Can you work these out from the model? Positions are in its coordinate system, mm. A direction names the side the tool comes from. Round coordinates to 2 decimals unless told otherwise and drop trailing zeros. Order: outer loops, then holes, each group sorted by start corner. A loop starts at its lowest first (then second) coordinate and runs counter-clockwise, first axis right, second up. Notation, with made-up numbers: (14, 23) -> (22, 23) arc R22 cw to (22, 58) -> close; hole circle Ø5 at (67, -35). An arc over 180 degrees is marked (long way). One line per item, written item: value.
```python
from build123d import *

# Parameters (mm, degrees)
BOSS_EXTRUDE1_DEPTH = 27
SKETCH3_R           = 1.7
CUT_EXTRUDE2_DEPTH  = 35.322004603
SKETCH4_W           = 10
SKETCH4_H           = 20
CUT_EXTRUDE3_DEPTH  = 1
SKETCH5_R           = 2.25
CUT_EXTRUDE4_DEPTH  = 36.057096286
BOSS_EXTRUDE2_DEPTH = 3
SKETCH7_W           = 7
SKETCH7_H           = 3
BOSS_EXTRUDE3_DEPTH = 27
SKETCH8_R           = 2.25
CUT_EXTRUDE5_DEPTH  = 59.446556785
SKETCH9_R           = 4.25
CUT_EXTRUDE6_DEPTH  = 59.446556785
SKETCH11_W          = 16
SKETCH11_H          = 9
CUT_EXTRUDE7_DEPTH  = 59.446556785


with BuildPart() as part:
    # Sketch1 → Boss-Extrude1 (new body)
    with BuildSketch(Plane.XY):
        Polygon((0, 0), (0, 20), (3, 20), (3, 0), (10, 0), (10, -3), (0, -3), align=None)
    extrude(amount=BOSS_EXTRUDE1_DEPTH)

    # Sketch3 → Cut-Extrude2 (cut, through all)
    with BuildSketch(Plane(origin=(3, 0, 0), x_dir=(0, 0, -1), z_dir=(1, 0, 0))):
        with Locations(Location((-22, 14.85, 0), (0, 0, 90))):
            Circle(SKETCH3_R)
        with Locations(Location((-3, 14.85, 0), (0, 0, 90))):
            Circle(SKETCH3_R)
    extrude(amount=-CUT_EXTRUDE2_DEPTH, mode=Mode.SUBTRACT)

    # Sketch4 → Cut-Extrude3 (cut)
    with BuildSketch(Plane(origin=(3, 0, 0), x_dir=(0, 0, -1), z_dir=(1, 0, 0))):
        with Locations((-12.5, 10)):
            Rectangle(SKETCH4_W, SKETCH4_H)
    extrude(amount=-CUT_EXTRUDE3_DEPTH, mode=Mode.SUBTRACT)

    # Sketch5 → Cut-Extrude4 (cut, through all)
    with BuildSketch(Plane(origin=(0, 0, 0), x_dir=(1, 0, 0), z_dir=(0, 1, 0))):
        with Locations(Location((6.5, -9, 0), (0, 0, 270))):
            Circle(SKETCH5_R)
    extrude(amount=-CUT_EXTRUDE4_DEPTH, mode=Mode.SUBTRACT)

    # Sketch6 → Boss-Extrude2 (add)
    with BuildSketch(Plane.ZY):
        Polygon((27, 9), (54, 0), (54, -3), (27, -3), align=None)
    extrude(amount=-BOSS_EXTRUDE2_DEPTH)

    # Sketch7 → Boss-Extrude3 (add)
    with BuildSketch(Plane.XY.offset(27)):
        with Locations((6.5, -1.5)):
            Rectangle(SKETCH7_W, SKETCH7_H)
    extrude(amount=BOSS_EXTRUDE3_DEPTH)

    # Sketch8 → Cut-Extrude5 (cut, through all)
    with BuildSketch(Plane(origin=(0, 0, 0), x_dir=(1, 0, 0), z_dir=(0, 1, 0))):
        with Locations(Location((6.5, -39, 0), (0, 0, 270))):
            Circle(SKETCH8_R)
    extrude(amount=-CUT_EXTRUDE5_DEPTH, mode=Mode.SUBTRACT)

    # Sketch9 → Cut-Extrude6 (cut, through all)
    with BuildSketch(Plane(origin=(0, 0, 0), x_dir=(1, 0, 0), z_dir=(0, 1, 0))):
        with Locations((6.5, -39)):
            Circle(SKETCH9_R)
    extrude(amount=CUT_EXTRUDE6_DEPTH, mode=Mode.SUBTRACT)

    # Sketch11 → Cut-Extrude7 (cut, through all)
    with BuildSketch(Plane(origin=(10, 0, 0), x_dir=(0, 0, -1), z_dir=(1, 0, 0))):
        with Locations((-8, 1.5)):
            Rectangle(SKETCH11_W, SKETCH11_H)
    extrude(amount=-CUT_EXTRUDE7_DEPTH, mode=Mode.SUBTRACT)


solid = part.part
```
Q1. I want a section at B-B on z = 3. List the corners of the cut face in (x, y) for me.
Answers below:
outline: (0, 6) -> (3, 6) -> (3, 13.15) -> (0, 13.15) -> close; (0, 16.55) -> (3, 16.55) -> (3, 20) -> (0, 20) -> close
Q2. I want a section at C-C on x = 6.5. List the corners of the cut face in (y, z) for me, plus the area to 4 significant figures.
Answers below:
outline: (-3, 16) -> (0, 16) -> (0, 36.75) -> (-3, 36.75) -> close; (-3, 41.25) -> (0, 41.25) -> (0, 54) -> (-3, 54) -> close
area: 100.5 mm^2
Q3. Please list where these lines run through material, in increasing order: line 1 along Z through (x, y) = (1.9, 14.85); line 2 along X through (y, z) = (-1.75, 39); line 3 along Z through (x, y) = (1, 15.5).
Answers below:
line 1: 0 to 1.3, 4.7 to 20.3, 23.7 to 27
line 2: 0 to 4.25, 8.75 to 10
line 3: 0 to 1.43, 4.57 to 20.43, 23.57 to 27
Q4. On a 3-axis mill with a long thin cutter (end or side, diameter ignored), from which of +Z, -Z, +X, -X, +Y, -Y can I reach the whole of each face in a straight line? I mean faces 5 (the face through (2, 15, 27)), 6 (the face through (2, 12, 13)), 7 (the face through (2.5, 12.9, 7.5)), 8 (the face through (4, -1, 16)). Say none if no direction works.
Answers below:
face 5: +Z, +X, -X, +Y
face 6: +X, +Y
face 7: +X, +Y, -Y
face 8: -Z, +X, -X, -Y
Q5. I want a section at A-A on y = 14.85. List the corners of the cut face in (x, z) for me, plus the area to 3 significant figures.
Answers below:
outline: (0, 0) -> (3, 0) -> (3, 1.3) -> (0, 1.3) -> close; (0, 4.7) -> (3, 4.7) -> (3, 7.5) -> (2, 7.5) -> (2, 17.5) -> (3, 17.5) -> (3, 20.3) -> (0, 20.3) -> close; (0, 23.7) -> (3, 23.7) -> (3, 27) -> (0, 27) -> close
area: 50.6 mm^2
Q6. Will these pins go through, and if not, where does the flat tip stop? pin 1 Ø4 at (y, z) = (15.5, 5) entering from +X; pin 2 Ø6 at (x, z) = (8.5, 37) entering from +Y; pin 3 Ø0.8 at (x, y) = (2.5, 14.5) entering from +Z.
Answers below:
pin 1: x = 3
pin 2: y = 0
pin 3: z = 27
Q7. We'd pull the mould along Y, two halves only. Please class faces 1 (the face through (3, 1, 45)), 2 (the face through (1.52, 13.6, 23.15)), 3 (the face through (1, 6, 8)), 4 (the face through (1.52, 13.15, 3.07)): released by +Y, released by -Y, zero draft, split by the parting line, or undercut.
Answers below:
face 1: zero draft
face 2: undercut
face 3: released by -Y
face 4: undercut
Q8. I want a section at D-D on z = 39. List the corners of the cut face in (x, y) for me, plus the area to 4 significant figures.
Answers below:
outline: (0, -3) -> (4.25, -3) -> (4.25, 0) -> (2.25, 0) -> (2.25, 5) -> (0, 5) -> close; (8.75, -3) -> (10, -3) -> (10, 0) -> (8.75, 0) -> close
area: 27.75 mm^2
